The figure shows three views and two pictorial views of one solid part (mm, origin at its lowest corner). Answer the questions. A direction names the side the tool comes from. Coordinates: 2 decimals unless noted, no trailing zeros. Order: outer loops, then holes, each group sorted by start corner. A loop starts at its lowest first (then second) coordinate and runs counter-clockwise, first axis right, second up.
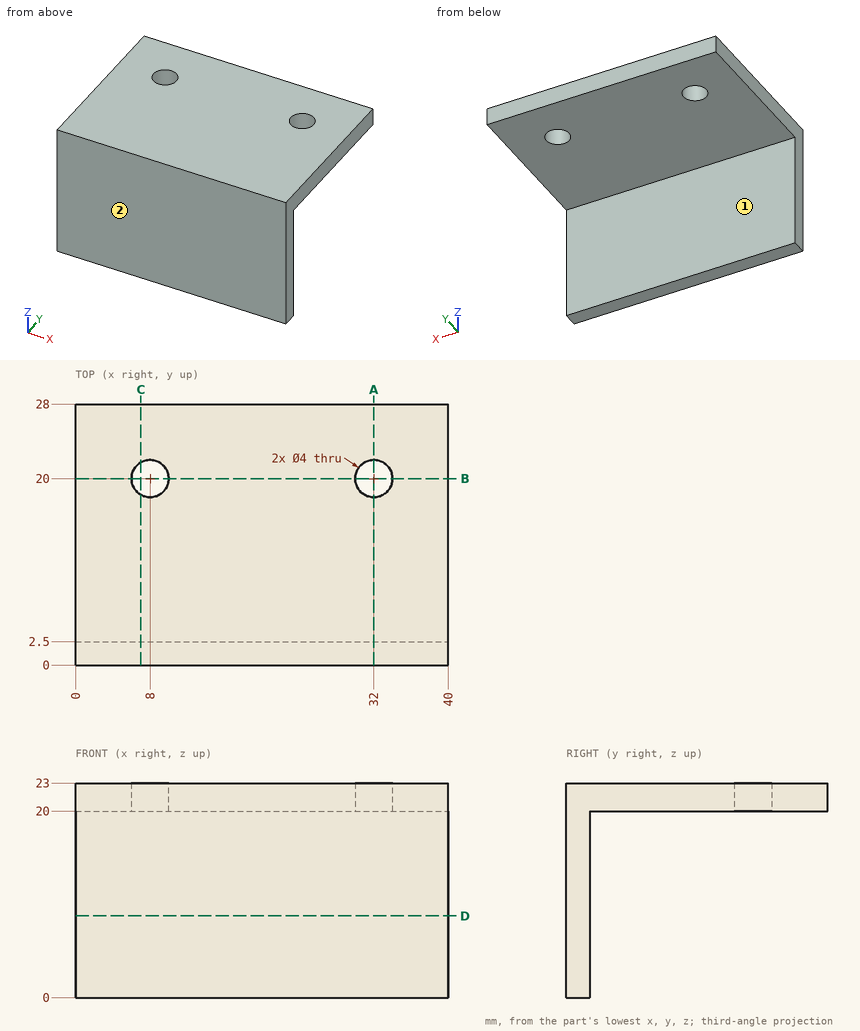
Q1. Straight lines are drawn through the part: L1, parallel to X at y = 20, z = 21.5; L2, parallel to Y at x = 8, z = 20.75; L3, parallel to Z at x = 29.5, y = 12.75. For each, find the intervals that lie inside material, in ascending order.
Q2. Each of these flat-tipped pins is pushed along its axis until it touches: P1, Ø6.5, axis at x = 8, y = 20, coming from the -Z side; P2, Ø3, axis at x = 32, z = 4, coming from the +Y side; P3, Ø5, axis at x = 12.5, z = 19, coming from the -Y side. Where does it stop, or does it pass through?
Q3. The part is cut by section C-C, the plane x = 7. Determine the outline of the cut face in (y, z), then the cut area to 3 significant figures.
Q4. Which of the six approach directions +Z, -Z, +X, -X, +Y, -Y give full straight-line access (tool end or side, diameter ignored) to the marked faces 1 and 2?
Q5. The part is cut by section A-A, the plane x = 32. Determine the outline of the cut face in (y, z), then the cut area to 3 significant figures.
Q6. The part is cut by section D-D, the plane z = 8.75. Determine the outline of the cut face in (x, y).
Q7. The part is cut by section B-B, the plane y = 20. Determine the outline of the cut face in (x, z).
Computed values:
1. L1: x = 0 to 6, 10 to 30, 34 to 40
1. L2: y = 0 to 18, 22 to 28
1. L3: z = 20 to 23
2. P1: stops at z = 20
2. P2: stops at y = 2.5
2. P3: stops at y = 0
3. outline: (0, 0) - (2.5, 0) - (2.5, 20) - (18.27, 20) - (18.27, 23) - (0, 23) - close; (21.73, 20) - (28, 20) - (28, 23) - (21.73, 23) - close
3. area: 124 mm2
4. face 1: -Z, +X, -X, +Y
4. face 2: +Z, -Z, +X, -X, -Y
5. outline: (0, 0) - (2.5, 0) - (2.5, 20) - (18, 20) - (18, 23) - (0, 23) - close; (22, 20) - (28, 20) - (28, 23) - (22, 23) - close
5. area: 122 mm2
6. outline: (0, 0) - (40, 0) - (40, 2.5) - (0, 2.5) - close
7. outline: (0, 20) - (6, 20) - (6, 23) - (0, 23) - close; (10, 20) - (30, 20) - (30, 23) - (10, 23) - close; (34, 20) - (40, 20) - (40, 23) - (34, 23) - close
